```python
from build123d import *

# Parameters (mm, degrees)
SKETCH1_W           = 150
SKETCH1_H           = 21.4
BOSS_EXTRUDE2_DEPTH = 2
SKETCH2_W           = 5
SKETCH2_H           = 2
BOSS_EXTRUDE3_DEPTH = 2.5
LPATTERN1_COUNT     = 15
LPATTERN1_PITCH     = 10
SKETCH3_W           = 5
SKETCH3_H           = 2
BOSS_EXTRUDE4_DEPTH = 2.5
LPATTERN2_COUNT     = 15
LPATTERN2_PITCH     = 10
CUT_EXTRUDE1_DEPTH  = 10


with BuildPart() as part:
    # Sketch1 → Boss-Extrude2 (new body)
    with BuildSketch(Plane.XY):
        with Locations((75, 10.7)):
            Rectangle(SKETCH1_W, SKETCH1_H)
    extrude(amount=BOSS_EXTRUDE2_DEPTH)

    # Sketch2 → Boss-Extrude3 (add)
    with BuildSketch(Plane(origin=(0, 21.4, 0), x_dir=(1, 0, 0), z_dir=(0, 1, 0))):
        with Locations((2.5, -1)):
            Rectangle(SKETCH2_W, SKETCH2_H)
    boss_extrude3 = extrude(amount=BOSS_EXTRUDE3_DEPTH)

    # LPattern1: Boss-Extrude3 ×15
    with Locations(*[(i * LPATTERN1_PITCH, 0, 0) for i in range(1, LPATTERN1_COUNT)]):
        add(boss_extrude3)

    # Sketch3 → Boss-Extrude4 (add)
    with BuildSketch(Plane(origin=(0, 0, 0), x_dir=(-1, 0, 0), z_dir=(0, -1, 0))):
        with Locations((-2.5, -1)):
            Rectangle(SKETCH3_W, SKETCH3_H)
    boss_extrude4 = extrude(amount=BOSS_EXTRUDE4_DEPTH)

    # LPattern2: Boss-Extrude4 ×15
    with Locations(*[(i * LPATTERN2_PITCH, 0, 0) for i in range(1, LPATTERN2_COUNT)]):
        add(boss_extrude4)

    # Sketch4 → Cut-Extrude1 (cut)
    with BuildSketch(Plane(origin=(0, 0, 0), x_dir=(-1, 0, 0), z_dir=(0, 0, -1))):
        with BuildLine():
            Line((-140, 6.45), (-90, 6.45))
            ThreePointArc((-90, 6.45), (-88.45, 4.9), (-90, 3.35))
            Line((-90, 3.35), (-140, 3.35))
            ThreePointArc((-140, 3.35), (-141.55, 4.9), (-140, 6.45))
        make_face()
        with BuildLine():
            Line((-45, 12.25), (-5, 12.25))
            ThreePointArc((-5, 12.25), (-3.45, 10.7), (-5, 9.15))
            Line((-5, 9.15), (-45, 9.15))
            ThreePointArc((-45, 9.15), (-46.55, 10.7), (-45, 12.25))
        make_face()
    extrude(amount=-CUT_EXTRUDE1_DEPTH, mode=Mode.SUBTRACT)


solid = part.part
```
Verification items for the finished model (mm, model axes). Coordinates: 2 decimals unless noted, no trailing zeros. Loops run counter-clockwise (first coordinate to the right, second up) from the corner with the lowest first, then second, coordinate; pieces in that order, holes last. Notation, with made-up numbers: (23.5, 48) -> (44.5, 48) arc R8 cw to (44.5, 53) -> close; hole circle Ø9 at (-28, 48). An arc over 180 degrees is marked (long way). Answer in a Markdown table with one row per item. Add a question column.
1. Section check A-A, the plane x = 68.5. Enter the section's corners in (y, z).
2. Section check B-B, the plane z = 1.7. Give the number of separate pieces and of enclosed holes in the cut face, then the cut area to 3 significant figures.
3. Depth check by flat-ended pin: P1, Ø1, axis at x = 118.5, z = 0.5, coming from the -Y side; P2, Ø0.6, axis at y = 22.5, z = 1, coming from the +X side. Enter the tip coordinate at first touch or a pass-through.
4. Material ranges on probe 1 along Y at (x, z) = (32, 1.6); probe 2 along Y at (x, z) = (128, 0.1); probe 3 along X at (y, z) = (10.5, 0.1), recorded low to high. Write a range as [from, to].
Derived:
| question | item | result |
|---|---|---|
| 1 | outline | (0, 0) -> (21.4, 0) -> (21.4, 2) -> (0, 2) -> close |
| 2 | separate pieces | 1 |
| 2 | enclosed holes | 2 |
| 2 | area | 3,290 mm² |
| 3 | P1 | stops at y = 0 |
| 3 | P2 | stops at x = 145 |
| 4 | probe 1 | y = [-2.5, 9.15], [12.25, 23.9] |
| 4 | probe 2 | y = [0, 3.35], [6.45, 21.4] |
| 4 | probe 3 | x = [0, 3.46], [46.54, 150] |
